Answer from the drawing. Dimensions are ordinates in mm from the lowest x, y and z of the part. Round coordinates to 2 decimals unless told otherwise and drop trailing zeros. Loops run counter-clockwise (first coordinate to the right, second up) from the corner with the lowest first, then second, coordinate; pieces in that order, holes last.
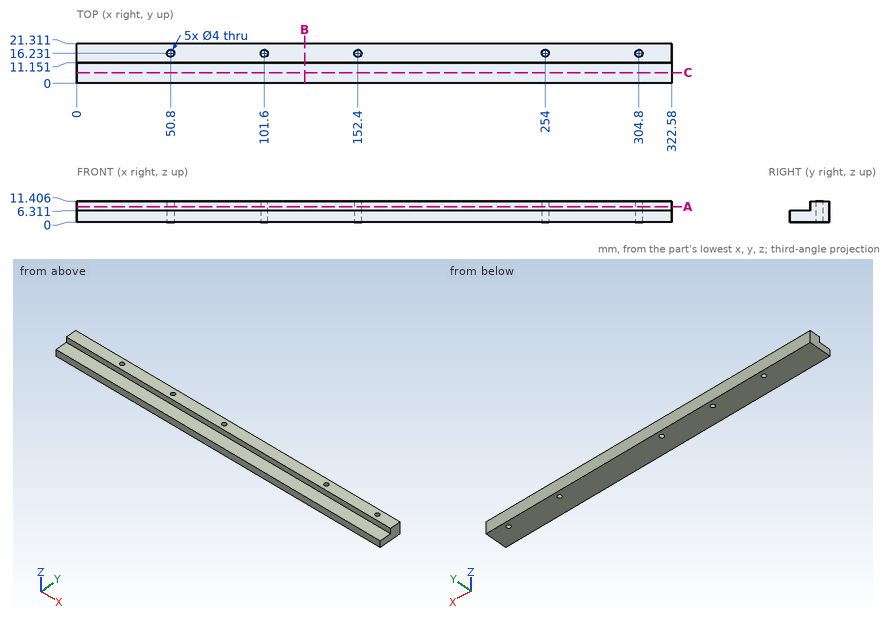
Item 1: Each of these flat-tipped pins is pushed along its axis until it touches: P1, Ø2.5, axis at x = 218, z = 10, coming from the -Y side; P2, Ø9, axis at x = 200, y = 4.5, coming from the +Z side. Where does it stop, or does it pass through?
Item 2: Straight lines are drawn through the part: line 1 (X direction, y = 16.5, z = 6.25); line 2 (X direction, y = 15.25, z = 9); line 3 (Y direction, x = 47, z = 10.75). For each, find the intervals that lie inside material, in ascending order.
Item 3: Section A-A, the plane z = 8.5 is taken. Give the vertices of the cut face in (x, y), plus the area to 3 significant figures.
Item 4: Section B-B, the plane x = 123.5 is taken. Give the vertices of the cut face in (y, z), plus the area to 3 significant figures.
Item 5: Section C-C, the plane y = 5.75 is taken. Give the vertices of the cut face in (x, z).
Answer below:
1. P1: stops at y = 11.15
1. P2: stops at z = 6.31
2. line 1: x = 0 to 48.82, 52.78 to 99.62, 103.58 to 150.42, 154.38 to 252.02, 255.98 to 302.82, 306.78 to 322.58
2. line 2: x = 0 to 49.06, 52.54 to 99.86, 103.34 to 150.66, 154.14 to 252.26, 255.74 to 303.06, 306.54 to 322.58
2. line 3: y = 11.15 to 21.31
3. outline: (0, 11.15) - (322.58, 11.15) - (322.58, 21.31) - (0, 21.31) - close; hole circle Ø4 at (50.8, 16.23); hole circle Ø4 at (101.6, 16.23); hole circle Ø4 at (152.4, 16.23); hole circle Ø4 at (254, 16.23); hole circle Ø4 at (304.8, 16.23)
3. area: 3,210 mm2
4. outline: (0, 0) - (21.31, 0) - (21.31, 11.41) - (11.15, 11.41) - (11.15, 6.31) - (0, 6.31) - close
4. area: 186 mm2
5. outline: (0, 0) - (322.58, 0) - (322.58, 6.31) - (0, 6.31) - close
